from build123d import *

# Parameters (mm, degrees)
F0_R     = 6
F1_DEPTH = 2
F2_SIZE2 = 2.5980762114
F2_SIZE  = 1.5
F4_R     = 2.35
F4_R_2   = 1.4
F5_DEPTH = 7
F6_R     = 1.2


# Not quite as in the source:
# - a fillet or chamfer that OpenCascade refuses, or shapes differently, is made with other operations: its cross-section is extruded or revolved along the edge and cut away or added


with BuildPart() as f1:
    # F0 (on Top) → F1 (new body)
    with BuildSketch(Plane.XY):
        Circle(F0_R)
    extrude(amount=F1_DEPTH)

    # F2
    f2_edges = [f1.edges().sort_by_distance(p)[0] for p in [
        (-6, 0, 0),
    ]]
    f2_side = f1.faces().sort_by_distance((-6, 0, 1))[0]
    chamfer(f2_edges, length=F2_SIZE, length2=F2_SIZE2, reference=f2_side)

    # F3: fillet of radius 1 on 2 edges, made by hand

    # F3_s1 → F3_t2 (revolve, cut)
    with BuildSketch(Plane.XZ):
        with BuildLine():
            ThreePointArc((3.6339745962, 0.1339745962), (3.3927936413, 0.0340741737), (3.1339745962, 0))
            Line((3.1339745962, 0), (3.4019237886, 0))
            Line((3.4019237886, 0), (3.6339745962, 0.1339745962))
        make_face()
    revolve(axis=Axis((0, 0, 0), (0, 0, 1)), mode=Mode.SUBTRACT)

    # F3_s3 → F3_t4 (revolve, cut)
    with BuildSketch(Plane.XZ):
        with BuildLine():
            ThreePointArc((6, 2), (5.8486778537, 1.5452494356), (5.5031382462, 1.2131367327))
            Line((5.5031382462, 1.2131367327), (6, 1.5))
            Line((6, 1.5), (6, 2))
        make_face()
    revolve(axis=Axis((0, 0, 1.5), (0, 0, 1)), mode=Mode.SUBTRACT)

    # F4 (on face) → F5 (join)
    with BuildSketch(Plane.XY.offset(2)):
        Circle(F4_R)
        Circle(F4_R_2, mode=Mode.SUBTRACT)
    extrude(amount=F5_DEPTH)

    # F6
    f6_edges = [f1.edges().sort_by_distance(p)[0] for p in [
        (-1.4, 0, 2),
    ]]
    fillet(f6_edges, radius=F6_R)


solid = f1.part
Build history of the part. All positions in model axes, mm. A direction names the side the tool comes from. Give positions to 0.01 mm unless a question says otherwise; leave off trailing zeros. Order: outer loops, then holes, each group sorted by start corner. A loop starts at its lowest first (then second) coordinate and runs counter-clockwise, first axis right, second up. Notation, with made-up numbers: M 89.25,-32.75 L 136.25,-32.75 A10 ccw 136.25,-16.75 Z; hole C -17,13.5 d5. An arc over 180 degrees is marked long. Put each result on its own line as item: value.
Item 1: Cut at A-A on z = 4.5. Write the cut outline in (x, y).
Results are:
outline: C 0,0 d4.7; hole C 0,0 d2.8
Item 2: Cut at B-B on z = 1.75. Write the cut outline in (x, y).
Results are:
outline: C 0,0 d11.89
Item 3: Which spindle directions (+Z, -Z, +X, -X, +Y, -Y) get a long thin tool onto all of the face, cutting with end or side? Do faces 1 (the face through (3, 0, 2)), 2 (the face through (0, -2, 9)). Say none if no direction does.
Results are:
face 1: +Z
face 2: +Z, +X, -X, +Y, -Y
Item 4: Wall check: probe 1 along Y at (x, z) = (0, 7.1); probe 2 along Y at (x, z) = (0.5, 7.75); probe 3 along Z at (x, y) = (-1, -2.25). Give the ranges that are in metal, low to high.
Results are:
probe 1: -2.35 to -1.4, 1.4 to 2.35
probe 2: -2.3 to -1.31, 1.31 to 2.3
probe 3: 0 to 2
Item 5: Pull direction X, two halves, no side cores. Call faces 3 (the face through (0, 0, 0)), 4 (the face through (-0.509, -2.294, 5.451)), 5 (the face through (-1.4, 0.06, 6.06)): +X half, -X half, draft (parallel to the pull), parting line (faces both ways), or undercut.
Results are:
face 3: draft
face 4: parting line
face 5: undercut
Item 6: Drop flat-ended pins along their axis: pin 1 Ø1.5 at (x, y) = (-1, 0) entering from -Z; pin 2 Ø2 at (x, z) = (-3.5, 7.5) entering from -Y; pin 3 Ø3 at (x, y) = (-4.5, 2.5) entering from -Z; pin 4 Ø1 at (y, z) = (0.5, 1.5) entering from -X. Give the stop position or say it passes through.
Results are:
pin 1: z = 0
pin 2: through
pin 3: z = 0.14
pin 4: x = -5.99
